from build123d import *

# Parameters (mm, degrees)
SKETCH1_W           = 101.6
SKETCH1_H           = 88.9
BOSS_EXTRUDE1_DEPTH = 3.175
SKETCH2_W           = 3.175
SKETCH2_H           = 12.7
BOSS_EXTRUDE2_DEPTH = 3.175
SKETCH3_R           = 1.65
CUT_EXTRUDE1_DEPTH  = 4.175


with BuildPart() as part:
    # Sketch1 → Boss-Extrude1 (new body)
    with BuildSketch(Plane.XY):
        with Locations((50.8, 44.45)):
            Rectangle(SKETCH1_W, SKETCH1_H)
    extrude(amount=BOSS_EXTRUDE1_DEPTH)

    # Sketch2 → Boss-Extrude2 (add)
    with BuildSketch(Plane.XY.offset(3.175)):
        with Locations((-1.5875, 44.45)):
            Rectangle(SKETCH2_W, SKETCH2_H)
        with Locations((103.1875, 44.45)):
            Rectangle(SKETCH2_W, SKETCH2_H)
    extrude(amount=-BOSS_EXTRUDE2_DEPTH)

    # Sketch3 → Cut-Extrude1 (cut, through all)
    with BuildSketch(Plane.XY.offset(3.175)):
        with Locations((27.589999938, 69.85)):
            Circle(SKETCH3_R)
        with Locations((75.790000058, 69.85)):
            Circle(SKETCH3_R)
        with Locations((62.19000008, 19.05)):
            Circle(SKETCH3_R)
        with Locations((34.29, 19.05)):
            Circle(SKETCH3_R)
    extrude(amount=-CUT_EXTRUDE1_DEPTH, mode=Mode.SUBTRACT)


solid = part.part
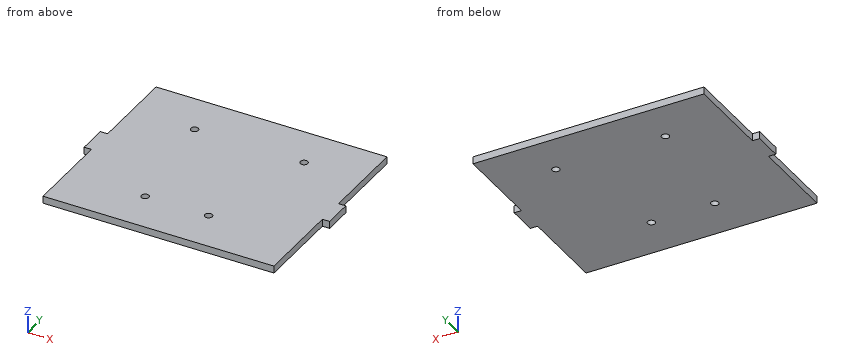
Can you work these out from the model? Positions are in its coordinate system, mm. Coordinates: 2 decimals unless noted, no trailing zeros. Write each loop counter-clockwise with the first axis right and the second up, starting at its lowest first coordinate (ties: lowest second). Pieces come first, ordered by that corner, then holes.
Q1. Please list where these lines run through material, in increasing order: L1, parallel to X at y = 69.85, z = 1.65; L2, parallel to Y at x = 34.29, z = 0.7; L3, parallel to X at y = 51, z = 2.6.
Results found:
L1: x = 0 to 25.94, 29.24 to 74.14, 77.44 to 101.6
L2: y = 0 to 17.4, 20.7 to 88.9
L3: x = 0 to 101.6
Q2. Imagine slicing it at B-B, the plane z = 2.55. List the corners of the cut face in (x, y) for me (3 decimals).
Results found:
outline: (-3.175, 38.1) - (0, 38.1) - (0, 0) - (101.6, 0) - (101.6, 38.1) - (104.775, 38.1) - (104.775, 50.8) - (101.6, 50.8) - (101.6, 88.9) - (0, 88.9) - (0, 50.8) - (-3.175, 50.8) - close; hole circle Ø3.3 at (27.59, 69.85); hole circle Ø3.3 at (34.29, 19.05); hole circle Ø3.3 at (62.19, 19.05); hole circle Ø3.3 at (75.79, 69.85)
Q3. Imagine slicing it at A-A, the plane x = 27.59. List the corners of the cut face in (y, z) for me (3 decimals).
Results found:
outline: (0, 0) - (68.2, 0) - (68.2, 3.175) - (0, 3.175) - close; (71.5, 0) - (88.9, 0) - (88.9, 3.175) - (71.5, 3.175) - close
Q4. Imagine slicing it at D-D, the plane y = 80. List the corners of the cut face in (x, z) for me (3 decimals), plus the area to 3 significant figures.
Results found:
outline: (0, 0) - (101.6, 0) - (101.6, 3.175) - (0, 3.175) - close
area: 323 mm2
Q5. For P1, Ø1, axis at y = 27, z = 1, coming from the -X side; P2, Ø1, axis at x = -2.5, z = 2, coming from the +Y side; P3, Ø1.6, axis at x = -1, z = 1, coming from the -Y side, each with a flat end and sliding along its axis, tell me the tip position at first contact or that it passes through.
Results found:
P1: stops at x = 0
P2: stops at y = 50.8
P3: stops at y = 38.1
Q6. Imagine slicing it at C-C, the plane y = 69.85. List the corners of the cut face in (x, z) for me (3 decimals).
Results found:
outline: (0, 0) - (25.94, 0) - (25.94, 3.175) - (0, 3.175) - close; (29.24, 0) - (74.14, 0) - (74.14, 3.175) - (29.24, 3.175) - close; (77.44, 0) - (101.6, 0) - (101.6, 3.175) - (77.44, 3.175) - close
